Here's how the part is built. I have some questions about the finished solid (model axes, mm). Face numbers are marked on the shaded views. A direction names the side the tool comes from. Give positions to 0.01 mm unless a question says otherwise; leave off trailing zeros. Write each loop counter-clockwise with the first axis right and the second up, starting at its lowest first coordinate (ties: lowest second). Pieces come first, ordered by that corner, then holes. Notation, with made-up numbers: (-38, -24) - (1, -24) arc R16 ccw to (1, 6) - close; hole circle Ø4 at (39.5, -5). An arc over 180 degrees is marked (long way). Use one line per item in the form item = value. Start each with the question number.
from build123d import *

# Parameters (mm, degrees)
ESQUISSE1_R             = 50.5
BOSS_EXTRU_1_DEPTH      = 15
ESQUISSE2_R             = 82.5
BOSS_EXTRU_2_DEPTH      = 10
ESQUISSE3_W             = 40.5
ESQUISSE3_H             = 42.5
ENL_V_MAT_EXTRU_1_DEPTH = 2
ESQUISSE4_W             = 10
ESQUISSE4_H             = 16
ENL_V_MAT_EXTRU_2_DEPTH = 6.3
ESQUISSE5_W             = 50
ESQUISSE5_H             = 90
BOSS_EXTRU_3_DEPTH      = 6
BOSS_EXTRU_4_DEPTH      = 6
ESQUISSE7_R             = 3.5
ENL_V_MAT_EXTRU_3_DEPTH = 10
ESQUISSE8_R             = 3.5
ENL_V_MAT_EXTRU_4_DEPTH = 6
ESQUISSE9_R             = 3.5
BOSS_EXTRU_5_DEPTH      = 6
ENL_V_START             = -6
ESQUISSE10_R            = 3.5
ENL_V_MAT_EXTRU_5_DEPTH = 6
ESQUISSE13_R            = 3.5
ENL_V_MAT_EXTRU_6_DEPTH = 10
ESQUISSE17_R            = 3.5
ENL_V_MAT_EXTRU_7_DEPTH = 6
ESQUISSE19_R            = 3.5
BOSS_EXTRU_8_DEPTH      = 6
CONG_1_R                = 10
CONG_1_OF_SYM_TRIE4_R   = 10


with BuildPart() as part:
    # Esquisse1 → Boss.-Extru.1 (new body)
    with BuildSketch(Plane(origin=(0, 0, 0), x_dir=(1, 0, 0), z_dir=(0, 1, 0))):
        with Locations(Location((0, 0, 0), (0, 0, 270))):
            Circle(ESQUISSE1_R)
    extrude(amount=BOSS_EXTRU_1_DEPTH)

    # Esquisse2 → Boss.-Extru.2 (add)
    with BuildSketch(Plane(origin=(0, 15, 0), x_dir=(1, 0, 0), z_dir=(0, 1, 0))):
        with Locations(Location((0, 0, 0), (0, 0, 270))):
            Circle(ESQUISSE2_R)
    extrude(amount=BOSS_EXTRU_2_DEPTH)

    # Esquisse3 → Enlèv. mat.-Extru.1 (cut)
    with BuildSketch(Plane(origin=(0, 25, 0), x_dir=(1, 0, 0), z_dir=(0, 1, 0))):
        with Locations((34.25, 0)):
            Rectangle(ESQUISSE3_W, ESQUISSE3_H)
    extrude(amount=-ENL_V_MAT_EXTRU_1_DEPTH, mode=Mode.SUBTRACT)

    # Esquisse4 → Enlèv. mat.-Extru.2 (cut)
    with BuildSketch(Plane(origin=(0, 23, 0), x_dir=(1, 0, 0), z_dir=(0, 1, 0))):
        with Locations((49.5, 0)):
            Rectangle(ESQUISSE4_W, ESQUISSE4_H)
    extrude(amount=-ENL_V_MAT_EXTRU_2_DEPTH, mode=Mode.SUBTRACT)

    # Esquisse5 → Boss.-Extru.3 (add)
    with BuildSketch(Plane.ZY.offset(-54.5)):
        with Locations((0, 70)):
            Rectangle(ESQUISSE5_W, ESQUISSE5_H)
        with BuildLine():
            ThreePointArc((25, 115), (0, 140), (-25, 115))
            Line((-25, 115), (25, 115))
        make_face()
    boss_extru_3 = extrude(amount=-BOSS_EXTRU_3_DEPTH)

    # Symétrie1: Boss.-Extru.3 across plane
    add(boss_extru_3.mirror(Plane(origin=(0, 0, 0), x_dir=(0, 0, 1), z_dir=(1, 0, 0))))

    # Esquisse6 → Boss.-Extru.4 (add)
    with BuildSketch(Plane.ZY.offset(-54.5)):
        with BuildLine():
            Line((66.9, 140), (0, 140))
            ThreePointArc((0, 140), (17.67766953, 132.67766953), (25, 115))
            Line((25, 115), (25, 100.126441606))
            Line((25, 100.126441606), (66.9, 100.126441606))
            Line((66.9, 100.126441606), (66.9, 140))
        make_face()
        with BuildLine():
            Line((66.9, 140), (66.9, 100.126441606))
            ThreePointArc((66.9, 100.126441606), (86.836779197, 120.063220803), (66.9, 140))
        make_face()
    extrude(amount=-BOSS_EXTRU_4_DEPTH)

    # Esquisse7 → Enlèv. mat.-Extru.3 (cut)
    with BuildSketch(Plane(origin=(60.5, 0, 0), x_dir=(0, 0, -1), z_dir=(1, 0, 0))):
        with Locations((-66.9, 120.063220803)):
            Circle(ESQUISSE7_R)
    extrude(amount=-ENL_V_MAT_EXTRU_3_DEPTH, mode=Mode.SUBTRACT)

    # Esquisse8 → Enlèv. mat.-Extru.4 (cut)
    with BuildSketch(Plane(origin=(60.5, 0, 0), x_dir=(0, 0, -1), z_dir=(1, 0, 0))):
        with Locations((0, 120.063220803)):
            Circle(ESQUISSE8_R)
    extrude(amount=-ENL_V_MAT_EXTRU_4_DEPTH, mode=Mode.SUBTRACT)

    # Esquisse9 → Boss.-Extru.5 (add)
    with BuildSketch(Plane.ZY.offset(60.5)):
        with BuildLine():
            Line((0, 140), (66.9, 140))
            ThreePointArc((66.9, 140), (86.836779197, 120.063220803), (66.9, 100.126441606))
            Line((66.9, 100.126441606), (25, 100.126441606))
            Line((25, 100.126441606), (25, 115))
            ThreePointArc((25, 115), (17.67766953, 132.67766953), (0, 140))
        make_face()
        with Locations(Location((66.9, 120.063220803, 0), (0, 0, 180))):
            Circle(ESQUISSE9_R, mode=Mode.SUBTRACT)
    extrude(amount=-BOSS_EXTRU_5_DEPTH)

    # Esquisse10 → Enlèv. mat.-Extru.5 (cut)
    with BuildSketch(Plane.ZY.offset(60.5).offset(ENL_V_START)):
        with Locations(Location((0, 120.063220803, 0), (0, 0, 180))):
            Circle(ESQUISSE10_R)
    extrude(amount=ENL_V_MAT_EXTRU_5_DEPTH, mode=Mode.SUBTRACT)

    # Esquisse13 → Enlèv. mat.-Extru.6 (cut)
    with BuildSketch(Plane.ZY.offset(60.5)):
        with Locations((0, 53.163220803)):
            Circle(ESQUISSE13_R)
    extrude(amount=-ENL_V_MAT_EXTRU_6_DEPTH, mode=Mode.SUBTRACT)

    # Esquisse17 → Enlèv. mat.-Extru.7 (cut)
    with BuildSketch(Plane.ZY.offset(60.5)):
        with Locations((0, 107.085063293)):
            Circle(ESQUISSE17_R)
    enl_v_mat_extru_7 = extrude(amount=-ENL_V_MAT_EXTRU_7_DEPTH, mode=Mode.SUBTRACT)

    # Esquisse19 → Boss.-Extru.8 (add)
    # profile 1 of 2: a face of its own
    with BuildSketch(Plane.ZY.offset(60.5)):
        with Locations((0, 61.406086298)):
            Circle(ESQUISSE19_R)
    # profile 2 of 2: a face of its own
    with BuildSketch(Plane.ZY.offset(60.5)):
        with BuildLine():
            Line((25, 46.888681), (71.2950306, 46.888681))
            Line((71.2950306, 46.888681), (71.2950306, 100.616913422))
            ThreePointArc((71.2950306, 100.616913422), (69.111156744, 100.249438968), (66.9, 100.126441606))
            Line((66.9, 100.126441606), (52.2950306, 100.126441606))
            Line((52.2950306, 100.126441606), (52.2950306, 65.888681))
            Line((52.2950306, 65.888681), (25, 65.888681))
            Line((25, 65.888681), (25, 46.888681))
        make_face()
        with Locations((61.7950306, 78.794182581)):
            Circle(ESQUISSE19_R, mode=Mode.SUBTRACT)
    boss_extru_8 = extrude(amount=-BOSS_EXTRU_8_DEPTH)

    # Congé1
    cong_1_edges = [part.edges().sort_by_distance(p)[0] for p in [
        (-57.5, 46.888681, 71.2950306),
    ]]
    fillet(cong_1_edges, radius=CONG_1_R)

    # Symétrie4: Enlèv. mat.-Extru.7, Boss.-Extru.8 across plane
    add(enl_v_mat_extru_7.mirror(Plane(origin=(0, 0, 0), x_dir=(0, 0, 1), z_dir=(1, 0, 0))), mode=Mode.SUBTRACT)
    add(boss_extru_8.mirror(Plane(origin=(0, 0, 0), x_dir=(0, 0, 1), z_dir=(1, 0, 0))))

    # Congé1 of Symétrie4
    cong_1_of_sym_trie4_edges = [part.edges().sort_by_distance(p)[0] for p in [
        (57.5, 46.888681, 71.2950306),
    ]]
    fillet(cong_1_of_sym_trie4_edges, radius=CONG_1_OF_SYM_TRIE4_R)


solid = part.part
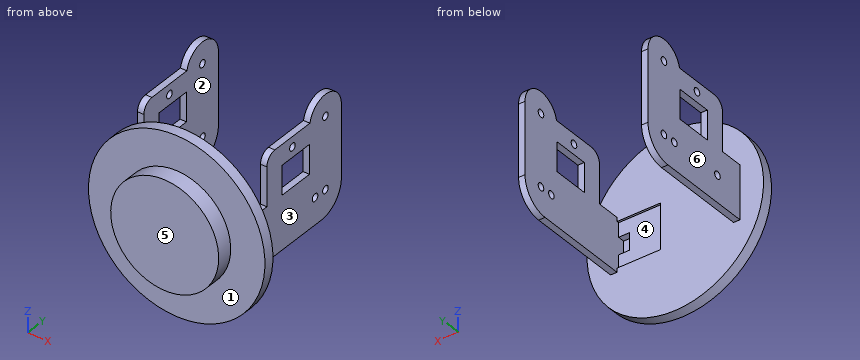
1. I want a section at C-C, the plane x = 0. List the corners of the cut face in (y, z) for me.
2. For the marked faces 1, 2 and 3, which set-ups out of +Z, -Z, +X, -X, +Y, -Y let a thin tool reach every point of the face, with its end or its side?
3. I want a section at A-A, the plane y = 60. List the corners of the cut face in (x, z) for me.
4. Please list where these lines run through material, in increasing order: line 1 (Y direction, x = -56, z = 0); line 2 (X direction, y = 61, z = 59); line 3 (Y direction, x = 45.5, z = -67).
5. For P1, Ø1.5, axis at y = 97, z = -25, coming from the -X side; P2, Ø1.6, axis at y = 24, z = 6, coming from the +X side; P3, Ø5, axis at x = 58.5, z = 49.5, coming from the -Y side, each with a flat end and sliding along its axis, tell me the tip position at first contact or that it passes through.
6. I want a section at B-B, the plane y = 91. List the corners of the cut face in (x, z) for me, then the cut area to 3 significant figures.
7. I want a section at D-D, the plane z = -31. List the corners of the cut face in (x, y) for me, then the cut area to 3 significant figures.
8. We'd pull the mould along X, two halves only. Please class the marked faces 4, 5 and 6: pulls with the +X half, pulls with the -X half, needs draft (parallel to the pull), parting line crosses it, or undercut.
Result sheet:
q1.outline = (0, -50.5) - (15, -50.5) - (15, -82.5) - (25, -82.5) - (25, 82.5) - (15, 82.5) - (15, 50.5) - (0, 50.5) - close
q2.face_1 = -Y
q2.face_2 = +Z, -Z, +Y
q2.face_3 = +Z, -Z, +X, +Y
q3.outline = (-60.5, -25) - (-54.5, -25) - (-54.5, 71.3) - (-60.5, 71.3) - close; (54.5, -25) - (60.5, -25) - (60.5, 71.3) - (54.5, 71.3) - close
q4.line_1 = 15 to 49.66, 56.66 to 103.59, 110.59 to 116.56, 123.56 to 140
q4.line_2 = -60.5 to -54.5, 54.5 to 60.5
q4.line_3 = 15 to 25
q5.P1 = -60.5
q5.P2 = 82.34
q5.P3 = 15
q6.outline = (-60.5, -25) - (-54.5, -25) - (-54.5, 25) - (-60.5, 25) - close; (-60.5, 52.3) - (-54.5, 52.3) - (-54.5, 71.3) - (-60.5, 71.3) - close; (54.5, -25) - (60.5, -25) - (60.5, 25) - (54.5, 25) - close; (54.5, 52.3) - (60.5, 52.3) - (60.5, 71.3) - (54.5, 71.3) - close
q6.area = 828 mm2
q7.outline = (-76.45, 15) - (-39.87, 15) - (-39.87, 0) - (39.87, 0) - (39.87, 15) - (76.45, 15) - (76.45, 25) - (-76.45, 25) - close
q7.area = 2,730 mm2
q8.face_4 = undercut
q8.face_5 = needs draft
q8.face_6 = pulls with the -X half
